Read the model definition and answer for the solid it produces. Units are mm, in the model's axes. Face numbers are marked on the shaded views. A direction names the side the tool comes from. Coordinates: 2 decimals unless noted, no trailing zeros. Write each loop counter-clockwise with the first axis right and the second up, starting at its lowest first coordinate (ties: lowest second). Pieces come first, ordered by that corner, then holes. Notation, with made-up numbers: (86.5, 74) - (125.5, 74) arc R6 cw to (125.5, 78) - close; hole circle Ø1 at (-1, 55). An arc over 180 degrees is marked (long way). Use a Markdown table: item, result.
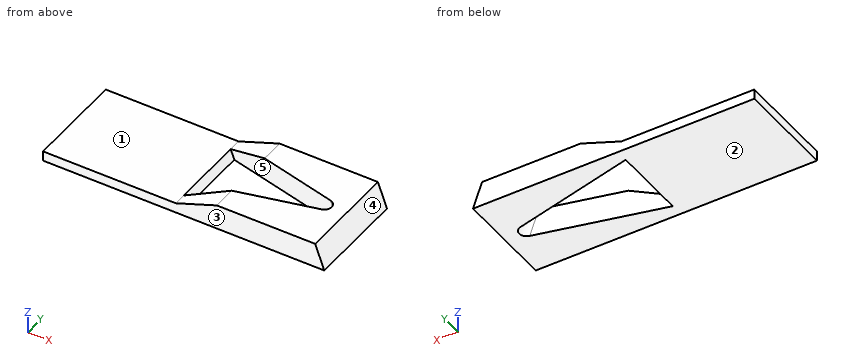
Autodesk Fusion 360 part; units mm, degrees
sketch "Sketch1" plane through (0, 0, 0) normal (0, 1, 0) x (1, 0, 0)
  line L0 (0, 0) -> (27, 0)
  line L1 (27, 0) -> (53, -9.4632)
  line L2 (53, -9.4632) -> (53, 0)
  line L3 (0, -2) -> (26.6473, -2)
  line L4 (26.6473, -2) -> (52.316, -11.3426)
  line L5 (53, -9.4632) -> (52.316, -11.3426)
  line L6 (0, -2) -> (0, 0)
  line L7 (53, 0) -> (27, 0)
  line L8 (53, -9.4632) -> (56.4443, 0)
  line L9 (56.4443, 0) -> (53, 0)
  dimension "d1" = 27
  dimension "d3" = 160
  dimension "d4" = 26
  dimension "d5" = 2
extrude "Extrude1" add sketch "Sketch1" along normal blind 20
sketch "Sketch2" plane through (2.4744, 0, -6.7982) normal (-0.342, 0, 0.9397) x (0, -1, 0)
  line L0 (0, 25.7244) -> (0, 53.0403)
  line L1 (0, 53.0403) -> (-20, 53.0403)
  line L2 (-20, 53.0403) -> (-20, 25.7244)
  line L3 (-20, 25.7244) -> (0, 25.7244)
  line L4 (-17.5, 25.7244) -> (-11.4522, 49.1091)
  line L5 (-8.5478, 49.1091) -> (-2.5, 25.7244)
  line L6 (-10, 25.7244) -> (-10, 53.0403)
  arc A0 (-8.5478, 49.1091) -> (-11.4522, 49.1091) centre (-10, 48.7335) ccw
  point P0 (-10, 54.7244)
  dimension "d8" = 7.5
  dimension "d9" = 7.5
  dimension "d10" = 29
  dimension "d11" = 1.5
extrude "Extrude2" cut sketch "Sketch2" against normal blind 15 contours L3 L5 L6 A0 | L3 L4 L6 A0
sketch "Sketch3" plane through (0, 20, 0) normal (0, 1, 0) x (-1, 0, 0)
  line L0 (-52.316, 11.3426) -> (-56.4443, 0)
  line L1 (-56.4443, 0) -> (0, 0)
  line L2 (0, 0) -> (0, 2)
  line L3 (0, 2) -> (-26.6473, 2)
  line L4 (-26.6473, 2) -> (-52.316, 11.3426)
  line L5 (-56.4443, 5) -> (-17.3231, 5)
  line L6 (-17.3231, 5) -> (-17.3231, 14.1022)
  line L7 (-17.3231, 14.1022) -> (-56.4443, 14.1022)
  line L8 (-56.4443, 14.1022) -> (-56.4443, 5)
  line L9 (-56.4443, 0) -> (-56.4443, 5)
  dimension "d14" = 5
extrude "Extrude3" cut sketch "Sketch3" against normal blind 86 contours L0 L4 L5 | L0 L4 L5 L6 L7 L8
equation "d9 = d8"
(1) A cutting plane is placed at A-A, the plane x = 33. Write down the section's boundary in (y, z), and give its area (3 significant figures).
Report:
| item | result |
|---|---|
| outline | (0, 0) - (3.87, 0) - (4.25, 4.31) - (0, 4.31) - close; (15.75, 4.31) - (16.13, 0) - (20, 0) - (20, 4.31) - close |
| area | 35.0 mm² |
(2) A cutting plane is placed at C-C, the plane y = 7. Write down the section's boundary in (x, z), and give its area (3 significant figures).
Report:
| item | result |
|---|---|
| outline | (0, 0) - (27.38, 0) - (26.65, 2) - (0, 2) - close; (44.07, 5) - (45.89, 0) - (56.44, 0) - (54.62, 5) - close |
| area | 107 mm² |
(3) The mould has two halves that part along Y. Classify the marked faces 3, 4 and 5: pulls with the +Y half, pulls with the -Y half, needs draft (parallel to the pull), parting line crosses it, or undercut.
Report:
| item | result |
|---|---|
| face 3 | pulls with the -Y half |
| face 4 | needs draft |
| face 5 | undercut |
(4) For the marked faces 1 and 2, determine the directions among +Z, -Z, +X, -X, +Y, -Y from which every point of the face is accessible in a straight line to the end or side of a thin tool.
Report:
| item | result |
|---|---|
| face 1 | +Z, -X, +Y, -Y |
| face 2 | -Z, +X, -X, +Y, -Y |
(5) A cutting plane is placed at D-D, the plane x = 10.5. Write down the section's boundary in (y, z), and give its area (3 significant figures).
Report:
| item | result |
|---|---|
| outline | (0, 0) - (20, 0) - (20, 2) - (0, 2) - close |
| area | 40.0 mm² |
(6) Each of these flat-tipped pins is pushed along its axis until it touches: P1, Ø1, axis at y = 5, z = 4, coming from the +X side; P2, Ø1.5, axis at y = 13.5, z = 1, coming from the +X side; P3, Ø10, axis at x = 16.5, y = 8.5, coming from the +Z side. Where does it stop, or does it pass through?
Report:
| item | result |
|---|---|
| P1 | stops at x = 55.17 |
| P2 | stops at x = 56.35 |
| P3 | stops at z = 2 |
(7) A cutting plane is placed at B-B, the plane y = 18.25. Write down the section's boundary in (x, z), and give its area (3 significant figures).
Report:
| item | result |
|---|---|
| outline | (0, 0) - (56.44, 0) - (54.62, 5) - (34.89, 5) - (26.65, 2) - (0, 2) - close |
| area | 185 mm² |
(8) Straight lines are drawn through the part: L1, parallel to Y at x = 41.5, z = 3.95; L2, parallel to Z at x = 8, y = 9.75; L3, parallel to Y at x = 45, z = 3.9. For each, find the intervals that lie inside material, in ascending order.
Report:
| item | result |
|---|---|
| L1 | y = 0 to 6.28, 13.72 to 20 |
| L2 | z = 0 to 2 |
| L3 | y = 0 to 7.13, 12.87 to 20 |
